```python
from build123d import *

# Parameters (mm, degrees)
F0_W        = 20.9
F0_H        = 9.5
F1_DEPTH    = 1.5
F2_W        = 16.9
F2_H        = 5.5
F3_DEPTH    = 1
F4_T1_DEPTH = 1
F5_T1_DEPTH = 26.5


# Not quite as in the source:
# - a fillet or chamfer that OpenCascade refuses, or shapes differently, is made with other operations: its cross-section is extruded or revolved along the edge and cut away or added


with BuildPart() as f1:
    # F0 (on Top) → F1 (new body)
    with BuildSketch(Plane.XY):
        with Locations((0.1440625638, -0.617788887)):
            Rectangle(F0_W, F0_H)
    extrude(amount=F1_DEPTH)

    # F2 (on Top) → F3 (cut)
    with BuildSketch(Plane.XY):
        with Locations((0.1440625638, -0.617788887)):
            Rectangle(F2_W, F2_H)
    extrude(amount=F3_DEPTH, mode=Mode.SUBTRACT)

    # F4: fillet of radius 3 on 4 edges, made by hand

    # F4_s2 → F4_t1 (join)
    with BuildSketch(Plane.XY):
        with BuildLine():
            ThreePointArc((8.5940625638, -0.367788887), (7.7153829073, -2.4891092305), (5.5940625638, -3.367788887))
            Line((5.5940625638, -3.367788887), (8.5940625638, -3.367788887))
            Line((8.5940625638, -3.367788887), (8.5940625638, -0.367788887))
        make_face()
        with BuildLine():
            ThreePointArc((-5.3059374362, 2.132211113), (-7.4272577798, 1.2535314566), (-8.3059374362, -0.867788887))
            Line((-8.3059374362, -0.867788887), (-8.3059374362, 2.132211113))
            Line((-8.3059374362, 2.132211113), (-5.3059374362, 2.132211113))
        make_face()
        with BuildLine():
            ThreePointArc((8.5940625638, -0.867788887), (7.7153829073, 1.2535314566), (5.5940625638, 2.132211113))
            Line((5.5940625638, 2.132211113), (8.5940625638, 2.132211113))
            Line((8.5940625638, 2.132211113), (8.5940625638, -0.867788887))
        make_face()
        with BuildLine():
            ThreePointArc((-8.3059374362, -0.367788887), (-7.4272577798, -2.4891092305), (-5.3059374362, -3.367788887))
            Line((-5.3059374362, -3.367788887), (-8.3059374362, -3.367788887))
            Line((-8.3059374362, -3.367788887), (-8.3059374362, -0.367788887))
        make_face()
    extrude(amount=F4_T1_DEPTH)

    # F5: fillet of radius 5 on 4 edges, made by hand

    # F5_s2 → F5_t1 (cut)
    with BuildSketch(Plane.XY.offset(-12.5)):
        with BuildLine():
            ThreePointArc((-10.3059374362, -0.867788887), (-8.8414713422, 2.667745019), (-5.3059374362, 4.132211113))
            Line((-5.3059374362, 4.132211113), (-10.3059374362, 4.132211113))
            Line((-10.3059374362, 4.132211113), (-10.3059374362, -0.867788887))
        make_face()
        with BuildLine():
            ThreePointArc((-5.3059374362, -5.367788887), (-8.8414713422, -3.9033227929), (-10.3059374362, -0.367788887))
            Line((-10.3059374362, -0.367788887), (-10.3059374362, -5.367788887))
            Line((-10.3059374362, -5.367788887), (-5.3059374362, -5.367788887))
        make_face()
        with BuildLine():
            ThreePointArc((10.5940625638, -0.867788887), (9.1295964697, 2.667745019), (5.5940625638, 4.132211113))
            Line((5.5940625638, 4.132211113), (10.5940625638, 4.132211113))
            Line((10.5940625638, 4.132211113), (10.5940625638, -0.867788887))
        make_face()
        with BuildLine():
            ThreePointArc((5.5940625638, -5.367788887), (9.1295964697, -3.9033227929), (10.5940625638, -0.367788887))
            Line((10.5940625638, -0.367788887), (10.5940625638, -5.367788887))
            Line((10.5940625638, -5.367788887), (5.5940625638, -5.367788887))
        make_face()
    extrude(amount=F5_T1_DEPTH, mode=Mode.SUBTRACT)


solid = f1.part
```
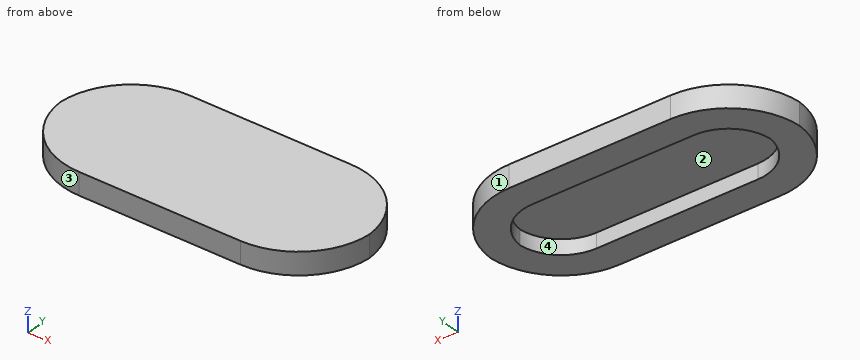
CAD build for the part. Positions are in the model's coordinates, mm. Face numbers are marked on the shaded views. Give positions to 0.01 mm unless a question says otherwise; leave off trailing zeros. Loops run counter-clockwise (first coordinate to the right, second up) from the corner with the lowest first, then second, coordinate; pieces in that order, holes last. Notation, with made-up numbers: (18, 66.25) - (55, 66.25) arc R8 ccw to (55, 79.25) - close; hole circle Ø6 at (58, 85). An arc over 180 degrees is marked (long way). Put each result on its own line as item: value.
Q1. Slice it at B-B (y = -2.5). Give the cut face in (x, z).
Filled in:
outline: (-9.83, 0) - (-7.42, 0) - (-7.42, 1) - (7.7, 1) - (7.7, 0) - (10.12, 0) - (10.12, 1.5) - (-9.83, 1.5) - close
Q2. Flat gauge pins, fed straight in: pin 1 (5 mm diameter, centred on x = 1, y = -1, fed in from -Z); pin 2 (3 mm diameter, centred on x = 0.5, y = 0.5, fed in from -Z). Where does each tip first touch, or does it go through?
Filled in:
pin 1: stops at z = 0
pin 2: stops at z = 1
Q3. Slice it at D-D (y = -5). Give the cut face in (x, z), plus the area to 3 significant figures.
Filled in:
outline: (-7.19, 0) - (7.48, 0) - (7.48, 1.5) - (-7.19, 1.5) - close
area: 22.0 mm²
Q4. Probe line 1 along Y through (x, z) = (4, 0.9); line 2 along Z through (x, y) = (-5.25, 1); line 3 along Y through (x, z) = (8.25, 0.25). List the from-to ranges inside material, lowest first.
Filled in:
line 1: y = -5.37 to -3.37, 2.13 to 4.13
line 2: z = 1 to 1.5
line 3: y = -4.6 to -1.76, 0.53 to 3.37
Q5. Mould opens along X. For the marked faces 1, 2, 3 and 4 say: pulls with the +X half, pulls with the -X half, needs draft (parallel to the pull), parting line crosses it, or undercut.
Filled in:
face 1: pulls with the +X half
face 2: undercut
face 3: pulls with the -X half
face 4: undercut
Q6. Slice it at C-C (x = 7.5). Give the cut face in (y, z).
Filled in:
outline: (-4.99, 0) - (-2.68, 0) - (-2.68, 1) - (1.45, 1) - (1.45, 0) - (3.75, 0) - (3.75, 1.5) - (-4.99, 1.5) - close
Q7. Slice it at A-A (z = 0.65). Give the cut face in (x, y), plus the area to 3 significant figures.
Filled in:
outline: (-10.3, -0.62) arc R5 ccw to (-5.31, -5.37) - (5.59, -5.37) arc R5 ccw to (10.59, -0.62) arc R5 ccw to (5.59, 4.13) - (-5.31, 4.13) arc R5 ccw to start; hole (-8.3, -0.62) arc R3 ccw to (-5.31, -3.37) - (5.59, -3.37) arc R3 ccw to (8.58, -0.62) arc R3 ccw to (5.59, 2.13) - (-5.31, 2.13) arc R3 ccw to start
area: 91.9 mm²
